from build123d import *

# Parameters (mm, degrees)
SKETCH1_R           = 1.1
BOSS_EXTRUDE1_DEPTH = 2


with BuildPart() as part:
    # Sketch1 → Boss-Extrude1 (new body)
    with BuildSketch(Plane.XY):
        with BuildLine():
            Line((5, -6.674), (-5, -6.674))
            Line((-5, -6.674), (-5, -8.674))
            Line((-5, -8.674), (-13, -8.674))
            Line((-13, -8.674), (-13, -6.674))
            Line((-13, -6.674), (-16, -6.674))
            Line((-16, -6.674), (-12.508255124, -2.282440657))
            ThreePointArc((-12.508255124, -2.282440657), (-12.346867401, -1.989679888), (-12.290989968, -1.660085322))
            Line((-12.290989968, -1.660085322), (-12.290989968, 1.65413052))
            ThreePointArc((-12.290989968, 1.65413052), (-12.235112536, 1.983725086), (-12.073724813, 2.276485855))
            Line((-12.073724813, 2.276485855), (-8, 7.4))
            Line((-8, 7.4), (-8, 2.4))
            Line((-8, 2.4), (-8, -0.6))
            Line((-8, -0.6), (-6, -0.6))
            Line((-6, -0.6), (-6, 2.4))
            Line((-6, 2.4), (6, 2.4))
            Line((6, 2.4), (6, -0.6))
            Line((6, -0.6), (8, -0.6))
            Line((8, -0.6), (8, 2.4))
            Line((8, 2.4), (8, 7.4))
            Line((8, 7.4), (12.073724813, 2.276485855))
            ThreePointArc((12.073724813, 2.276485855), (12.235112536, 1.983725086), (12.290989968, 1.65413052))
            Line((12.290989968, 1.65413052), (12.290989968, -1.660085322))
            ThreePointArc((12.290989968, -1.660085322), (12.346867401, -1.989679888), (12.508255124, -2.282440657))
            Line((12.508255124, -2.282440657), (16, -6.674))
            Line((16, -6.674), (13, -6.674))
            Line((13, -6.674), (13, -8.674))
            Line((13, -8.674), (5, -8.674))
            Line((5, -8.674), (5, -6.674))
        make_face()
        Circle(SKETCH1_R, mode=Mode.SUBTRACT)
    extrude(amount=BOSS_EXTRUDE1_DEPTH)


solid = part.part
Source: CAD feature listing. Evaluate the final solid. Frame: model axes, mm. A direction names the side the tool comes from. Round coordinates to 2 decimals unless told otherwise and drop trailing zeros. Write each loop counter-clockwise with the first axis right and the second up, starting at its lowest first coordinate (ties: lowest second). Pieces come first, ordered by that corner, then holes. Notation, with made-up numbers: (-11.75, 10.25) - (6.25, 10.25) arc R20 ccw to (6.25, 24.25) - close; hole circle Ø10 at (64, 29). An arc over 180 degrees is marked (long way). Use CSV: the item, a comma, the result in double quotes. Start each with the question number.
(1) Cut plane B-B, the plane x = 0. Return loops of the section in (y, z), and give its area (3 significant figures).
(2) First-contact query: pin 1 Ø1 at (x, z) = (-7, 1.5) entering from +Y; pin 2 Ø1 at (y, z) = (-7.5, 0.5) entering from +X; pin 3 Ø1 at (x, z) = (0, 1) entering from -Y. Flat tips, straight axial feed; report the tip coordinate or a pass-through.
(3) Material intervals for probe 1 along X at (y, z) = (1.75, 1.45); probe 2 along Y at (x, z) = (0, 0.85); probe 3 along X at (y, z) = (-7.25, 0.35), sorted ascending. Write a range as [from, to].
(4) Mould query, pull axis X, two halves, no side actions, for faces 4 (the face through (0, 2.4, 1)), 5 (the face through (-7, -0.6, 1)), 6 (the face through (-9, -8.674, 1)), 7 (the face through (-12.291, 0, 1)). Classes: pulls with the +X half, pulls with the -X half, needs draft (parallel to the pull), parting line crosses it, or undercut.
(5) Set-up query: faces 1 (the face through (6, 1, 1)), 2 (the face through (15, -6.674, 1)), 3 (the face through (-14, -6.674, 1)). Return all of +Z, -Z, +X, -X, +Y, -Y with unobstructed straight access to the full face (end or side cutting, diameter ignored); none if empty.
(6) Cut plane C-C, the plane y = 0. Return loops of the section in (x, z).
(7) Cut plane D-D, the plane z = 1.4. Return loops of the section in (x, y).
(8) Cut plane A-A, the plane y = -7.5. Return loops of the section in (x, z), and give its area (3 significant figures).
Geometry says:
1,outline,"(-6.67, 0) - (-1.1, 0) - (-1.1, 2) - (-6.67, 2) - close; (1.1, 0) - (2.4, 0) - (2.4, 2) - (1.1, 2) - close"
1,area,"13.7 mm²"
2,pin 1,"y = -0.6"
2,pin 2,"x = 13"
2,pin 3,"y = -6.67"
3,probe 1,"[-12.29, -8], [-6, 6], [8, 12.29]"
3,probe 2,"[-6.67, -1.1], [1.1, 2.4]"
3,probe 3,"[-13, -5], [5, 13]"
4,face 4,"undercut"
4,face 5,"undercut"
4,face 6,"needs draft"
4,face 7,"pulls with the -X half"
5,face 1,"+Z, -Z, +Y"
5,face 2,"+Z, -Z, +X, -Y"
5,face 3,"+Z, -Z, -X, -Y"
6,outline,"(-12.29, 0) - (-8, 0) - (-8, 2) - (-12.29, 2) - close; (-6, 0) - (-1.1, 0) - (-1.1, 2) - (-6, 2) - close; (1.1, 0) - (6, 0) - (6, 2) - (1.1, 2) - close; (8, 0) - (12.29, 0) - (12.29, 2) - (8, 2) - close"
7,outline,"(-16, -6.67) - (-13, -6.67) - (-13, -8.67) - (-5, -8.67) - (-5, -6.67) - (5, -6.67) - (5, -8.67) - (13, -8.67) - (13, -6.67) - (16, -6.67) - (12.51, -2.28) arc R1 cw to (12.29, -1.66) - (12.29, 1.65) arc R1 ccw to (12.07, 2.28) - (8, 7.4) - (8, -0.6) - (6, -0.6) - (6, 2.4) - (-6, 2.4) - (-6, -0.6) - (-8, -0.6) - (-8, 7.4) - (-12.07, 2.28) arc R1 ccw to (-12.29, 1.65) - (-12.29, -1.66) arc R1 cw to (-12.51, -2.28) - close; hole circle Ø2.2 at (0, 0)"
8,outline,"(-13, 0) - (-5, 0) - (-5, 2) - (-13, 2) - close; (5, 0) - (13, 0) - (13, 2) - (5, 2) - close"
8,area,"32.0 mm²"
